The listing builds one solid part. Answer for the finished solid, in the listing's coordinates (mm). A direction names the side the tool comes from. Give positions to 0.01 mm unless a question says otherwise; leave off trailing zeros. Order: outer loops, then holes, each group sorted by start corner. A loop starts at its lowest first (then second) coordinate and runs counter-clockwise, first axis right, second up. Notation, with made-up numbers: M -1.75,-5 L 45.25,-5 A22 ccw 45.25,2 Z; hole C -5.75,65 d2. An arc over 180 degrees is marked long. Answer as a JSON object with one key per item and string values. Group by question number.
```python
from build123d import *

# Parameters (mm, degrees)
F1_DEPTH = 25.4
F2_R     = 5.08
F3_DEPTH = 12.7
F4_R     = 5.08
F5_DEPTH = 6.351


with BuildPart() as f1:
    # F0 (on Top) → F1 (new body)
    with BuildSketch(Plane.XY):
        Polygon((-20.574, 6.35), (-82.55, 6.35), (-82.55, -82.55), (6.35, -82.55), (6.35, -20.574), (0, -20.574), (0, -76.2), (-76.2, -76.2), (-76.2, 0), (-20.574, 0), align=None)
    extrude(amount=F1_DEPTH)

    # F2 (on face) → F3 (cut)
    with BuildSketch(Plane.XZ):
        with Locations((-29.464, 12.7)):
            Circle(F2_R)
    extrude(amount=-F3_DEPTH, mode=Mode.SUBTRACT)

    # F4 (on face) → F5 (cut, through all)
    with BuildSketch(Plane(origin=(0, 0, 0), x_dir=(0, -1, 0), z_dir=(-1, 0, 0))):
        with Locations((29.464, 12.7)):
            Circle(F4_R)
    extrude(amount=-F5_DEPTH, mode=Mode.SUBTRACT)


solid = f1.part
```
Item 1: Section C-C (z = 12.7) is taken. Determine the outline of the cut face in (x, y), and give its area (3 significant figures).
Item 2: A tool of negligible diameter and unlimited length cuts with its end or side. For faces 5 (the flat face through (-38, -76.2, 13)), 6 (the cylindrical face through (3.131, -28.803, 17.737)), 7 (the flat face through (3, -20.574, 13)), 8 (the flat face through (-78, -44, 25.4)), 9 (the cylindrical face through (-24.62, 3.13, 14.23)), from which of +Z, -Z, +X, -X, +Y, -Y can it reach the whole face along a straight path? Write none if from no direction.
Item 3: Section A-A (y = -67) is taken. Determine the outline of the cut face in (x, z), and give its area (3 significant figures).
Item 4: Consider probe 1 along X at (y, z) = (-40, 19.5); probe 2 along Y at (x, z) = (-6, 8). Determine where each line is inside the solid, lowest interval first. Write a range as from..to.
Item 5: Section D-D (z = 19) is taken. Determine the outline of the cut face in (x, y), and give its area (3 significant figures).
Item 6: Flat-ended cylindrical pins translate along their axes: P1, Ø5, axis at y = 3, z = 16.5, coming from the +X side; P2, Ø12, axis at x = -70, y = -71.5, coming from the -Z side; P3, Ø5, axis at x = 3, z = 12, coming from the +Y side. Find the tip coordinate at first contact, or state that the pin passes through.
Item 7: Determine the mould class of faces 1 (the flat face through (-20.574, 3, 13)), 2 (the flat face through (0, -48, 13)), 3 (the flat face through (-49, 0, 13)), 4 (the flat face through (-82.55, -37, 13)) for opening direction X: released by +X, released by -X, zero draft, split by the parting line, or undercut.
Values found:
{
 "1": {"outline": "M -82.55,-82.55 L 6.35,-82.55 L 6.35,-34.54 L 0,-34.54 L 0,-76.2 L -76.2,-76.2 L -76.2,0 L -34.54,0 L -34.54,6.35 L -82.55,6.35 Z; M -24.38,0 L -20.57,0 L -20.57,6.35 L -24.38,6.35 Z; M 0,-24.38 L 6.35,-24.38 L 6.35,-20.57 L 0,-20.57 Z", "area": "1,670 mm^2"},
 "2": {"face 5": "+Z, -Z", "face 6": "+X", "face 7": "+Z, -Z, +X, +Y", "face 8": "+Z, +X, -X, +Y, -Y", "face 9": "+Y"},
 "3": {"outline": "M -82.55,0 L -76.2,0 L -76.2,25.4 L -82.55,25.4 Z; M 0,0 L 6.35,0 L 6.35,25.4 L 0,25.4 Z", "area": "323 mm^2"},
 "4": {"probe 1": "x = -82.55..-76.2, 0..6.35", "probe 2": "y = -82.55..-76.2"},
 "5": {"outline": "M -82.55,-82.55 L 6.35,-82.55 L 6.35,-20.57 L 0,-20.57 L 0,-76.2 L -76.2,-76.2 L -76.2,0 L -20.57,0 L -20.57,6.35 L -82.55,6.35 Z", "area": "1,800 mm^2"},
 "6": {"P1": "stops at x = -20.57", "P2": "stops at z = 0", "P3": "stops at y = -20.57"},
 "7": {"face 1": "released by +X", "face 2": "undercut", "face 3": "zero draft", "face 4": "released by -X"}
}
